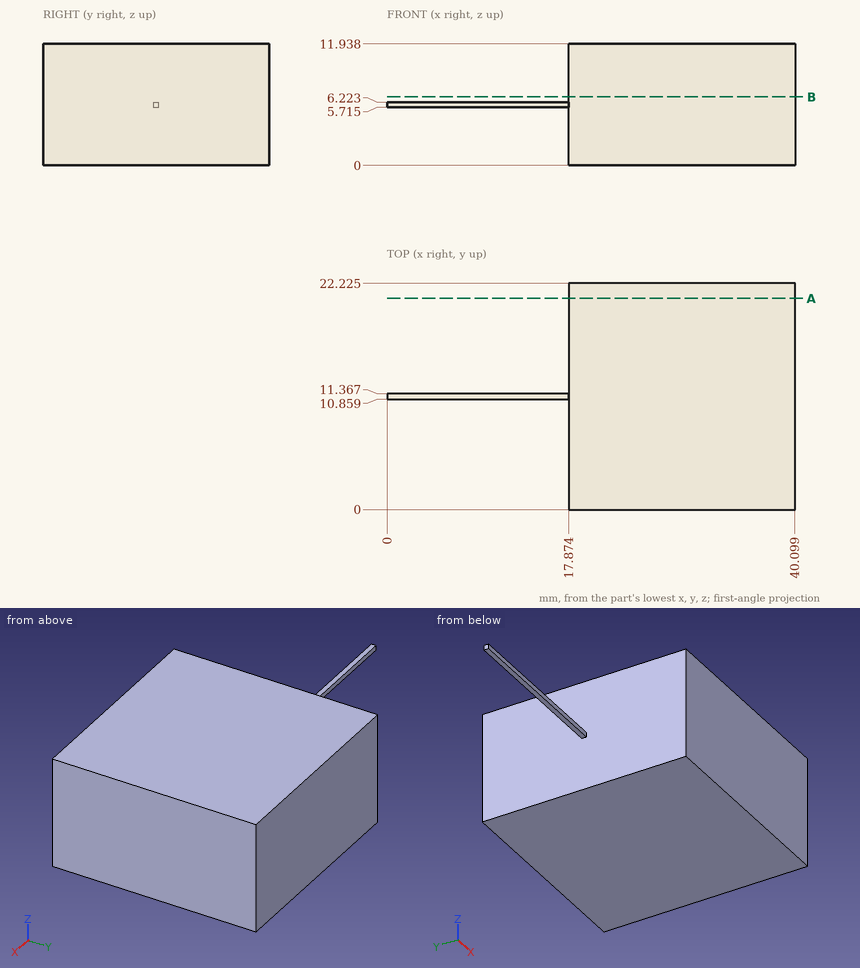
Answer from the drawing. Dimensions are ordinates in mm from the lowest x, y and z of the part. Round coordinates to 2 decimals unless told otherwise and drop trailing zeros. Write each loop counter-clockwise with the first axis right and the second up, starting at its lowest first coordinate (ties: lowest second). Pieces come first, ordered by that corner, then holes. Notation, with made-up numbers: (-32.5, 88.5) - (-16.5, 88.5) arc R33 ccw to (-16.5, 126.5) - close; hole circle Ø10 at (46.25, 37). An arc over 180 degrees is marked (long way). Use a Markdown table: item, result.
(1) Each of these flat-tipped pins is pushed along its axis until it touches: pin 1 Ø1 at (x, z) = (36, 1.5) entering from -Y; pin 2 Ø4 at (x, z) = (8, 8) entering from -Y; pin 3 Ø0.6 at (x, y) = (7.5, 11) entering from -Z (1 decimal); pin 4 Ø0.6 at (x, y) = (11.5, 11) entering from +Z. Where does it stop, or does it pass through?
Reported:
| item | result |
|---|---|
| pin 1 | y = 0 |
| pin 2 | y = 10.86 |
| pin 3 | z = 5.7 |
| pin 4 | z = 6.22 |
(2) The part is cut by section A-A (y = 20.75). Write down the section's boundary in (x, z) (1 decimal).
Reported:
| item | result |
|---|---|
| outline | (17.9, 0) - (40.1, 0) - (40.1, 11.9) - (17.9, 11.9) - close |
(3) A straight line is drawn through the part: line 1 along X through (y, z) = (10, 4) (1 decimal). Find the intervals that lie inside material, in ascending order. Write a range as [from, to].
Reported:
| item | result |
|---|---|
| line 1 | [17.9, 40.1] |
(4) The part is cut by section B-B (z = 6.75). Write down the section's boundary in (x, y) (1 decimal).
Reported:
| item | result |
|---|---|
| outline | (17.9, 0) - (40.1, 0) - (40.1, 22.2) - (17.9, 22.2) - close |
